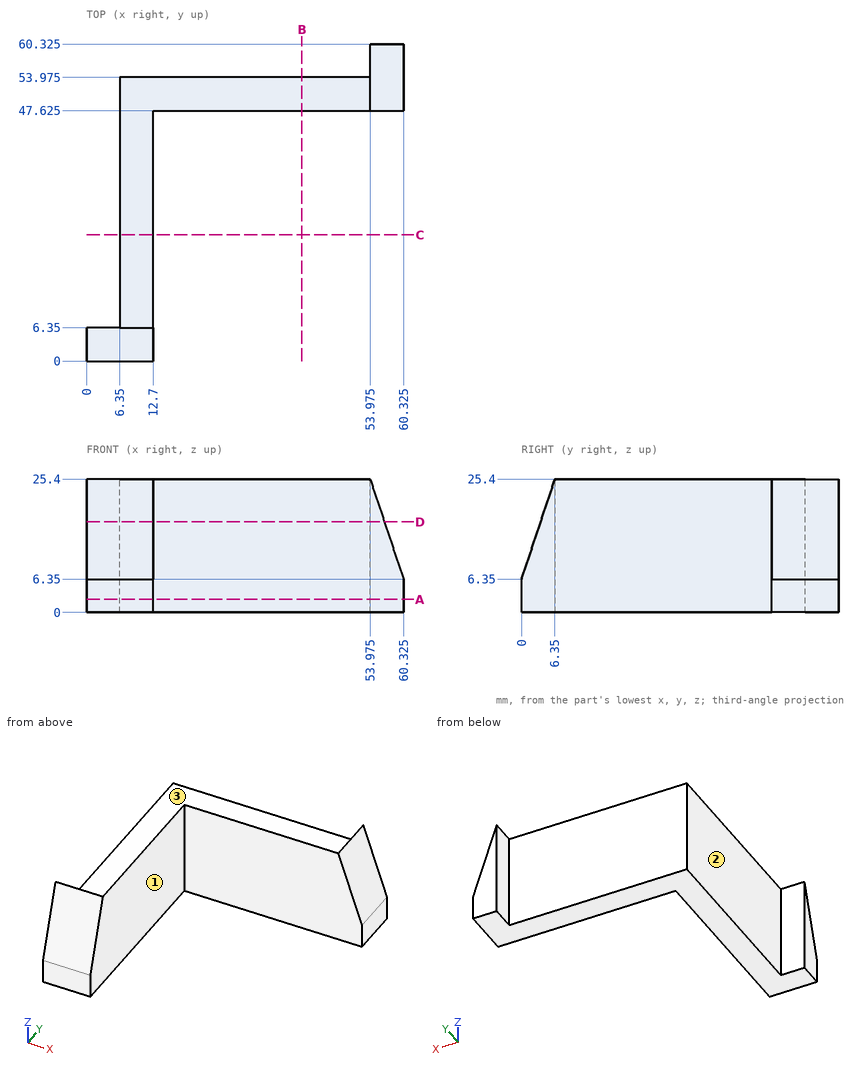
Geometry check sheet. Reference: drawing and pictorial views, mm from the part's lowest x, y, z. A direction names the side the tool comes from. Round coordinates to 2 decimals unless told otherwise and drop trailing zeros. Order: outer loops, then holes, each group sorted by start corner. A loop starts at its lowest first (then second) coordinate and runs counter-clockwise, first axis right, second up.
Q1. Cross-section at C-C, the plane y = 24. Enter the section's corners in (x, z), plus the area to 3 significant figures.
Filled sheet:
outline: (6.35, 0) - (12.7, 0) - (12.7, 25.4) - (6.35, 25.4) - close
area: 161 mm2
Q2. Depth check by flat-ended pin: P1, Ø7, axis at y = 56, z = 8.5, coming from the -X side; P2, Ø5, axis at y = 19, z = 4.5, coming from the +X side; P3, Ø1, axis at x = 42.5, z = 9.5, coming from the +Y side (3 decimals). Enter the tip coordinate at first touch or a pass-through.
Filled sheet:
P1: stops at x = 6.35
P2: stops at x = 12.7
P3: stops at y = 53.975
Q3. Cross-section at B-B, the plane x = 41. Enter the section's corners in (y, z) (3 decimals), plus the area to 3 significant figures.
Filled sheet:
outline: (47.625, 0) - (53.975, 0) - (53.975, 25.4) - (47.625, 25.4) - close
area: 161 mm2
Q4. Cross-section at D-D, the plane z = 17.25. Enter the section's corners in (x, y) (3 decimals), plus the area to 3 significant figures.
Filled sheet:
outline: (0, 3.633) - (12.7, 3.633) - (12.7, 47.625) - (56.692, 47.625) - (56.692, 60.325) - (53.975, 60.325) - (53.975, 53.975) - (6.35, 53.975) - (6.35, 6.35) - (0, 6.35) - close
area: 634 mm2
Q5. Scan lines: L1, parallel to X at y = 24, z = 17.75; L2, parallel to Y at x = 19.5, z = 7.75 (3 decimals); L3, parallel to Y at x = 4, z = 6.5. Record each from-to range of solid material in increasing order.
Filled sheet:
L1: x = 6.35 to 12.7
L2: y = 47.625 to 53.975
L3: y = 0.05 to 6.35
Q6. Set-up check for the marked faces 1, 2 and 3: record each of +Z, -Z, +X, -X, +Y, -Y from which the full face is reachable in a straight line by a thin tool's end or side.
Filled sheet:
face 1: +Z, -Z, +X, -Y
face 2: +Z, -Z, -X, +Y
face 3: +Z, +X, -X, +Y, -Y
Q7. Cross-section at A-A, the plane z = 2.5. Enter the section's corners in (x, y) (3 decimals), plus the area to 3 significant figures.
Filled sheet:
outline: (0, 0) - (12.7, 0) - (12.7, 47.625) - (60.325, 47.625) - (60.325, 60.325) - (53.975, 60.325) - (53.975, 53.975) - (6.35, 53.975) - (6.35, 6.35) - (0, 6.35) - close
area: 726 mm2
